from build123d import *

# Parameters (mm, degrees)
F0_W     = 76.2
F0_H     = 50.8
F1_DEPTH = 60
F2_R     = 7.62
F3_DEPTH = 76.201
F4_DEPTH = 76.201


with BuildPart() as f1:
    # F0 (on Front) → F1 (new body)
    with BuildSketch(Plane.XZ):
        with Locations((38.1, 25.4)):
            Rectangle(F0_W, F0_H)
        Polygon((38.1, 88.9), (0, 50.8), (76.2, 50.8), align=None)
    extrude(amount=F1_DEPTH)

    # F2 (on face) → F3 (cut, through all)
    with BuildSketch(Plane(origin=(0, 0, 0), x_dir=(0, -1, 0), z_dir=(-1, 0, 0))):
        with Locations((12.7, 20.32)):
            Circle(F2_R)
    extrude(amount=-F3_DEPTH, mode=Mode.SUBTRACT)

    # F2 (on face) → F4 (cut, through all)
    with BuildSketch(Plane(origin=(0, 0, 0), x_dir=(0, -1, 0), z_dir=(-1, 0, 0))):
        with Locations((12.7, 20.32)):
            Circle(F2_R)
        with Locations((38.1, 20.32)):
            Circle(F2_R)
    extrude(amount=-F4_DEPTH, mode=Mode.SUBTRACT)


solid = f1.part
Geometry: final body of the model. Coordinates: model frame, mm. Round coordinates to 2 decimals unless told otherwise and drop trailing zeros. Loops run counter-clockwise (first coordinate to the right, second up) from the corner with the lowest first, then second, coordinate; pieces in that order, holes last. Notation, with made-up numbers: (18.5, 25) -> (65.5, 25) arc R5 cw to (65.5, 29) -> close; hole circle Ø1 at (-31, 72). An arc over 180 degrees is marked (long way). One line per question, with ' | ' between items. Start each with the question number.
1. Section D-D on z = 80.5. Output: boundary loops of the cut face in (x, y).
2. Contact query for flat-ended pins moving along their axis: pin 1 (6 mm diameter, centred on y = -16.5, z = 78, fed in from -X); pin 2 (1.5 mm diameter, centred on x = 20, y = -21.5, fed in from +Z); pin 3 (8 mm diameter, centred on x = 9.5, y = -21, fed in from +Z). Output: stop coordinate, or through.
3. Line query: line 1 along Y through (x, z) = (43, 21); line 2 along Y through (x, z) = (23, 24.5); line 3 along Z through (x, y) = (37, -37). Output: solid intervals per line, ascending. Write a range as [from, to].
4. Mould query, pull axis Y, two halves, no side actions, for faces 1 (the face through (37.567, -32.053, 15.683)), 2 (the face through (38, 0, 35)), 3 (the face through (0, -30, 25)). Classes: pulls with the +Y half, pulls with the -Y half, needs draft (parallel to the pull), parting line crosses it, or undercut.
5. Section B-B on y = -12.7. Output: boundary loops of the cut face in (x, z).
6. Section A-A on z = 20.32. Output: boundary loops of the cut face in (x, y), and give its area (3 significant figures).
7. Section C-C on x = 57. Output: boundary loops of the cut face in (y, z), and give its area (3 significant figures).
Returned:
1) outline: (29.7, -60) -> (46.5, -60) -> (46.5, 0) -> (29.7, 0) -> close
2) pin 1: stops at x = 24.2 | pin 2: stops at z = 71.55 | pin 3: stops at z = 64.3
3) line 1: y = [-60, -45.69], [-30.51, -20.29], [-5.11, 0] | line 2: y = [-60, -44.47], [-31.73, -19.07], [-6.33, 0] | line 3: z = [0, 12.78], [27.86, 87.8]
4) face 1: undercut | face 2: pulls with the +Y half | face 3: needs draft
5) outline: (0, 0) -> (76.2, 0) -> (76.2, 12.7) -> (0, 12.7) -> close; (0, 27.94) -> (76.2, 27.94) -> (76.2, 50.8) -> (38.1, 88.9) -> (0, 50.8) -> close
6) outline: (0, -60) -> (76.2, -60) -> (76.2, -45.72) -> (0, -45.72) -> close; (0, -30.48) -> (76.2, -30.48) -> (76.2, -20.32) -> (0, -20.32) -> close; (0, -5.08) -> (76.2, -5.08) -> (76.2, 0) -> (0, 0) -> close | area: 2,250 mm2
7) outline: (-60, 0) -> (0, 0) -> (0, 70) -> (-60, 70) -> close; hole circle Ø15.24 at (-38.1, 20.32); hole circle Ø15.24 at (-12.7, 20.32) | area: 3,840 mm2
